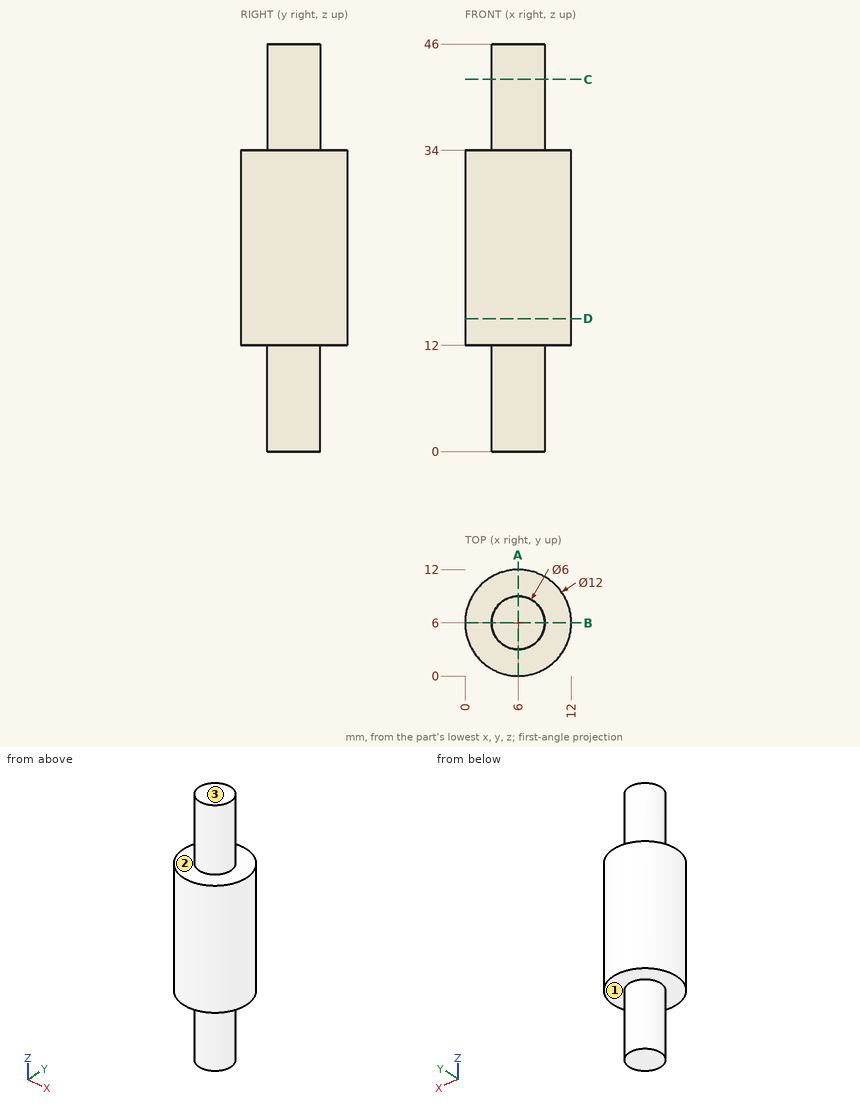
Can you work these out from the drawing? Everything is in mm from the part's minimum corner. A direction names the side the tool comes from. Give positions to 0.01 mm unless a question says otherwise; leave off trailing zeros. Order: outer loops, then holes, each group sorted by start corner. A loop starts at its lowest first (then second) coordinate and runs counter-clockwise, first axis right, second up. Notation, with made-up numbers: (-17, -35.75) -> (31, -35.75) arc R26 ccw to (31, -21.75) -> close; hole circle Ø2 at (-21, 14.25). An arc over 180 degrees is marked (long way). Return JSON: item names as keys, results as strings.
1. Imagine slicing it at A-A on x = 6. List the corners of the cut face in (y, z) for me, then the cut area to 3 significant figures.
Answer list:
{"outline": "(0, 12) -> (3, 12) -> (3, 0) -> (9, 0) -> (9, 12) -> (12, 12) -> (12, 34) -> (9, 34) -> (9, 46) -> (3, 46) -> (3, 34) -> (0, 34) -> close", "area": "408 mm2"}
2. Imagine slicing it at C-C on z = 42. List the corners of the cut face in (x, y) for me.
Answer list:
{"outline": "circle Ø6 at (6, 6)"}
3. I need wall thicknesses on line 1 (X direction, y = 6.25, z = 9); line 2 (Z direction, x = 4.25, y = 8.5); line 3 (X direction, y = 4.25, z = 6). Which ranges of each line are inside material? Lowest first, please. Write a range as from..to.
Answer list:
{"line 1": "x = 3.01..8.99", "line 2": "z = 12..34", "line 3": "x = 3.56..8.44"}
4. Imagine slicing it at D-D on z = 15. List the corners of the cut face in (x, y) for me, then the cut area to 3 significant figures.
Answer list:
{"outline": "circle Ø12 at (6, 6)", "area": "113 mm2"}
5. For pin 1 Ø1 at (x, y) = (3, 10.5) entering from +Z; pin 2 Ø6 at (x, z) = (6.5, 8) entering from +Y; pin 3 Ø1.5 at (x, z) = (3, 21) entering from +Y, each with a flat end and sliding along its axis, tell me the tip position at first contact or that it passes through.
Answer list:
{"pin 1": "stops at z = 34", "pin 2": "stops at y = 9", "pin 3": "stops at y = 11.56"}
6. On a 3-axis mill with a long thin cutter (end or side, diameter ignored), from which of +Z, -Z, +X, -X, +Y, -Y can I reach the whole of each face in a straight line? I mean the marked faces 1, 2 and 3. Say none if no direction works.
Answer list:
{"face 1": "-Z", "face 2": "+Z", "face 3": "+Z, +X, -X, +Y, -Y"}
